```python
from build123d import *

# Parameters (mm, degrees)
SKETCH1_W               = 120
SKETCH1_H               = 80
BOSS_EXTRUDE1_DEPTH     = 2
CUT_EXTRUDE1_DEPTH      = 20
CUT_EXTRUDE1_DEPTH_BACK = 20
SKETCH2_W               = 19
SKETCH2_H               = 22
CUT_EXTRUDE2_DEPTH      = 20
CUT_EXTRUDE2_DEPTH_BACK = 20
SKETCH3_W               = 19
SKETCH3_H               = 22
CUT_EXTRUDE3_DEPTH      = 20
CUT_EXTRUDE3_DEPTH_BACK = 20
SKETCH4_R               = 2


with BuildPart() as part:
    # Sketch1 → Boss-Extrude1 (new body)
    with BuildSketch(Plane(origin=(0, 0, 0), x_dir=(1, 0, 0), z_dir=(0, 1, 0))):
        Rectangle(SKETCH1_W, SKETCH1_H)
    extrude(amount=BOSS_EXTRUDE1_DEPTH)

    # Sketch2 → Cut-Extrude1 (cut, two sides: drawn at the far end of the back side and taken through both)
    with BuildSketch(Plane(origin=(0, 2, 0), x_dir=(1, 0, 0), z_dir=(0, 1, 0)).offset(-CUT_EXTRUDE1_DEPTH_BACK)):
        with Locations((-50.5, 0)):
            Rectangle(SKETCH2_W, SKETCH2_H)
    extrude(amount=CUT_EXTRUDE1_DEPTH + CUT_EXTRUDE1_DEPTH_BACK, mode=Mode.SUBTRACT)

    # Sketch3 → Cut-Extrude2 (cut, two sides: drawn at the far end of the back side and taken through both)
    with BuildSketch(Plane(origin=(0, 2, 0), x_dir=(1, 0, 0), z_dir=(0, 1, 0)).offset(-CUT_EXTRUDE2_DEPTH_BACK)):
        with Locations((50.5, 0)):
            Rectangle(SKETCH3_W, SKETCH3_H)
    extrude(amount=CUT_EXTRUDE2_DEPTH + CUT_EXTRUDE2_DEPTH_BACK, mode=Mode.SUBTRACT)

    # Sketch4 → Cut-Extrude3 (cut, two sides: drawn at the far end of the back side and taken through both)
    with BuildSketch(Plane(origin=(0, 2, 0), x_dir=(1, 0, 0), z_dir=(0, 1, 0)).offset(-CUT_EXTRUDE3_DEPTH_BACK)):
        with Locations(Location((-57, 37, 0), (0, 0, 90))):
            Circle(SKETCH4_R)
        with Locations(Location((57, 37, 0), (0, 0, 90))):
            Circle(SKETCH4_R)
        with Locations(Location((57, -37, 0), (0, 0, 90))):
            Circle(SKETCH4_R)
        with Locations(Location((-57, -37, 0), (0, 0, 90))):
            Circle(SKETCH4_R)
    extrude(amount=CUT_EXTRUDE3_DEPTH + CUT_EXTRUDE3_DEPTH_BACK, mode=Mode.SUBTRACT)


solid = part.part
```
Input: part model. Units: mm. Frame: model coordinates. Give positions to 0.01 mm unless a question says otherwise; leave off trailing zeros. Order: outer loops, then holes, each group sorted by start corner. A loop starts at its lowest first (then second) coordinate and runs counter-clockwise, first axis right, second up. Notation, with made-up numbers: (8, 84.5) - (34, 84.5) arc R12 ccw to (34, 106.5) - close; hole circle Ø5 at (-29.75, -3). An arc over 180 degrees is marked (long way). One line per item, written item: value.
1. Cut plane D-D, the plane y = 1.7. Output: boundary loops of the cut face in (x, z).
Determined:
outline: (-60, -40) - (60, -40) - (60, -11) - (41, -11) - (41, 11) - (60, 11) - (60, 40) - (-60, 40) - (-60, 11) - (-41, 11) - (-41, -11) - (-60, -11) - close; hole circle Ø4 at (-57, -37); hole circle Ø4 at (-57, 37); hole circle Ø4 at (57, -37); hole circle Ø4 at (57, 37)
2. Line query: probe 1 along X at (y, z) = (0.5, -37); probe 2 along Z at (x, y) = (-51, 1.9); probe 3 along X at (y, z) = (0.75, 1.5). Output: solid intervals per line, ascending.
Determined:
probe 1: -60 to -59, -55 to 55, 59 to 60
probe 2: -40 to -11, 11 to 40
probe 3: -41 to 41
3. Pin query (flat end, axial travel): pin 1 Ø1 at (y, z) = (1, 3.5) entering from -X. Return the tip coordinate at first contact, or that it passes through.
Determined:
pin 1: x = -41
4. Cut plane B-B, the plane z = 37. Output: boundary loops of the cut face in (x, y), and give its area (3 significant figures).
Determined:
outline: (-60, 0) - (-59, 0) - (-59, 2) - (-60, 2) - close; (-55, 0) - (55, 0) - (55, 2) - (-55, 2) - close; (59, 0) - (60, 0) - (60, 2) - (59, 2) - close
area: 224 mm2
5. Draft query along X for faces 1 (the face through (-59, 1, -37)), 2 (the face through (-1, 2, -1)), 3 (the face through (-59, 1, 37)). Return one class per face: released by +X, released by -X, zero draft, split by the parting line, or undercut.
Determined:
face 1: undercut
face 2: zero draft
face 3: undercut
6. Cut plane C-C, the plane x = -47.5. Output: boundary loops of the cut face in (y, z), and give its area (3 significant figures).
Determined:
outline: (0, -40) - (2, -40) - (2, -11) - (0, -11) - close; (0, 11) - (2, 11) - (2, 40) - (0, 40) - close
area: 116 mm2
7. Cut plane A-A, the plane x = 57. Output: boundary loops of the cut face in (y, z).
Determined:
outline: (0, -40) - (2, -40) - (2, -39) - (0, -39) - close; (0, -35) - (2, -35) - (2, -11) - (0, -11) - close; (0, 11) - (2, 11) - (2, 35) - (0, 35) - close; (0, 39) - (2, 39) - (2, 40) - (0, 40) - close
